```python
from build123d import *

# Parameters (mm, degrees)
SCHIZZO1_W                   = 20
SCHIZZO1_H                   = 20
ESTRUSIONE_ESTRUSIONE1_DEPTH = 58.2
SCHIZZO2_R                   = 2.05
TAGLIO_ESTRUSIONE1_DEPTH     = 60.893572276
FORO_FILETTATO_G1_8_1_D      = 8.8
FORO_FILETTATO_G1_8_1_DEPTH  = 10
FORO_FILETTATO_G1_8_1_TIP    = 2.643786724
M3_TAPPED_HOLE2_D            = 2.5
M3_TAPPED_HOLE2_DEPTH        = 5
M3_TAPPED_HOLE2_TIP          = 0.751075774
M3_TAPPED_HOLE3_REACH        = 60.911
M3_TAPPED_HOLE3_BORE_R       = 1.25
SKETCH1_W                    = 36.2
SKETCH1_H                    = 6
BOSS_EXTRUDE1_DEPTH          = 4.9
CUT_EXTRUDE1_DEPTH           = 65.087830449
M3_TAPPED_HOLE4_D            = 2.5
M3_TAPPED_HOLE4_DEPTH        = 20
M3_TAPPED_HOLE4_TIP          = 0.751075774


with BuildPart() as part:
    # Schizzo1 → Estrusione-Estrusione1 (new body)
    with BuildSketch(Plane.XY):
        Rectangle(SCHIZZO1_W, SCHIZZO1_H)
    extrude(amount=-ESTRUSIONE_ESTRUSIONE1_DEPTH)

    # Schizzo2 → Taglio-Estrusione1 (cut, through all)
    with BuildSketch(Plane(origin=(0, 0, -58.2), x_dir=(-1, 0, 0), z_dir=(0, 0, -1))):
        Circle(SCHIZZO2_R)
    extrude(amount=-TAGLIO_ESTRUSIONE1_DEPTH, mode=Mode.SUBTRACT)

    # Foro filettato G1/8-1
    with Locations(Plane.XY):
        with Locations((0, 0)):
            Hole(FORO_FILETTATO_G1_8_1_D / 2, depth=FORO_FILETTATO_G1_8_1_DEPTH)
            with Locations((0, 0, -(FORO_FILETTATO_G1_8_1_DEPTH + FORO_FILETTATO_G1_8_1_TIP / 2))):  # 118° drill point
                Cone(0, FORO_FILETTATO_G1_8_1_D / 2, FORO_FILETTATO_G1_8_1_TIP, mode=Mode.SUBTRACT)

    # M3 Tapped Hole2
    with Locations(Plane(origin=(0, 10, -29.1), x_dir=(1, 0, 0), z_dir=(0, 1, 0))):
        with Locations((0, 0)):
            Hole(M3_TAPPED_HOLE2_D / 2, depth=M3_TAPPED_HOLE2_DEPTH)
            with Locations((0, 0, -(M3_TAPPED_HOLE2_DEPTH + M3_TAPPED_HOLE2_TIP / 2))):  # 118° drill point
                Cone(0, M3_TAPPED_HOLE2_D / 2, M3_TAPPED_HOLE2_TIP, mode=Mode.SUBTRACT)

    # Schizzo14 → Foro Ø16.0 (16)-1 (revolve, cut)
    with BuildSketch(Plane(origin=(0, 0, -58.2), x_dir=(0, 1, 0), z_dir=(1, 0, 0))):
        Polygon((0, 0), (0, 16.806884952), (8, 12), (8, 0), align=None)
    revolve(axis=Axis((0, 0, -64.55), (0, 0, 1)), mode=Mode.SUBTRACT)

    # M3 Tapped Hole3 bore (on position points) → M3 Tapped Hole3 (cut, up to next)
    with BuildSketch(Plane(origin=(10, 5.5, -53.2), x_dir=(0, 0, 1), z_dir=(1, 0, 0)), mode=Mode.PRIVATE) as m3_tapped_hole3_sk1:
        Circle(M3_TAPPED_HOLE3_BORE_R)
    m3_tapped_hole3_tool1 = extrude(m3_tapped_hole3_sk1.sketch, amount=-M3_TAPPED_HOLE3_REACH, mode=Mode.PRIVATE) & part.part
    # M3 Tapped Hole3 bore (on position points) → M3 Tapped Hole3 (cut, up to next)
    with BuildSketch(Plane(origin=(10, 5.5, -53.2), x_dir=(0, 0, 1), z_dir=(1, 0, 0)), mode=Mode.PRIVATE) as m3_tapped_hole3_sk2:
        with Locations((0, 11)):
            Circle(M3_TAPPED_HOLE3_BORE_R)
    m3_tapped_hole3_tool2 = extrude(m3_tapped_hole3_sk2.sketch, amount=-M3_TAPPED_HOLE3_REACH, mode=Mode.PRIVATE) & part.part
    add(m3_tapped_hole3_tool1.solids().sort_by_distance((10, 5.5, -53.2))[0], mode=Mode.SUBTRACT)
    add(m3_tapped_hole3_tool2.solids().sort_by_distance((10, -5.5, -53.2))[0], mode=Mode.SUBTRACT)

    # Sketch1 → Boss-Extrude1 (add)
    with BuildSketch(Plane.ZY.offset(10)):
        with Locations((-40.1, 0)):
            Rectangle(SKETCH1_W, SKETCH1_H)
    extrude(amount=BOSS_EXTRUDE1_DEPTH)

    # Sketch2 → Cut-Extrude1 (cut, through all)
    with BuildSketch(Plane(origin=(10, 0, 0), x_dir=(0, 0, -1), z_dir=(1, 0, 0))):
        Polygon((50.1, -10), (34.1, -10), (8.1, -10), (8.1, -7), (34.1, -7), (50.1, -7), align=None)
    extrude(amount=-CUT_EXTRUDE1_DEPTH, mode=Mode.SUBTRACT)

    # M3 Tapped Hole4
    with Locations(Plane.XY.offset(-22)):
        with Locations((-13, 0)):
            Hole(M3_TAPPED_HOLE4_D / 2, depth=M3_TAPPED_HOLE4_DEPTH)
            with Locations((0, 0, -(M3_TAPPED_HOLE4_DEPTH + M3_TAPPED_HOLE4_TIP / 2))):  # 118° drill point
                Cone(0, M3_TAPPED_HOLE4_D / 2, M3_TAPPED_HOLE4_TIP, mode=Mode.SUBTRACT)


solid = part.part
```
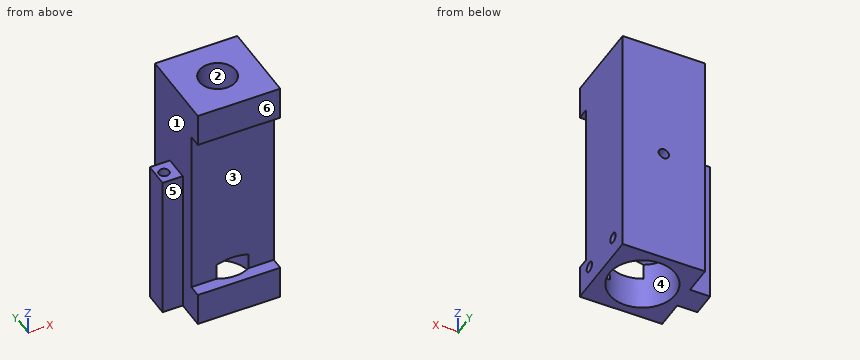
For this review, take the finished solid that the model builds, in its own axes (mm). Face numbers are marked on the shaded views. A direction names the side the tool comes from. Give positions to 0.01 mm unless a question says otherwise; leave off trailing zeros. Write each loop counter-clockwise with the first axis right and the second up, starting at its lowest first coordinate (ties: lowest second). Pieces come first, ordered by that corner, then holes. Notation, with made-up numbers: M -35,54 L -22,54 A23 ccw -22,73 Z; hole C -12.5,43 d9. An arc over 180 degrees is marked long. One line per item, written item: value.
1) For P1, Ø5, axis at x = 5.5, z = -45.5, coming from the -Y side; P2, Ø2, axis at y = -5.5, z = -53.2, coming from the +X side; P3, Ø1.5, axis at x = -11.5, y = -1, coming from the +Z side, all flat-tipped, find the tip position at first contact; note any pin that passes through.
Results are:
P1: stops at y = -7
P2: stops at x = -4.66
P3: stops at z = -22
2) Take a section at B-B, the plane z = -53.2. Write out the cut boundary in (x, y), then the cut area to 3 significant figures.
Results are:
outline: M -14.9,-3 L -10,-3 L -10,-10 L 10,-10 L 10,-6.75 L 4.29,-6.75 A8 cw long 4.29,6.75 L 10,6.75 L 10,10 L -10,10 L -10,3 L -14.9,3 Z; M 6.78,-4.25 L 10,-4.25 L 10,4.25 L 6.78,4.25 A8 cw Z
area: 207 mm²
3) Take a section at A-A, the plane z = -39. Write out the cut boundary in (x, y), then the cut area to 3 significant figures.
Results are:
outline: M -14.9,-3 L -10,-3 L -10,-7 L 10,-7 L 10,10 L -10,10 L -10,3 L -14.9,3 Z; hole C -13,0 d2.5; hole C 0,0 d4.1
area: 351 mm²
4) For the marked faces 4, 5 and 6, list the 3-axis set-ups (+Z, -Z, +X, -X, +Y, -Y) from which the entire face can be reached by the end or side of a thin tool; tool diameter is ignored.
Results are:
face 4: -Z
face 5: +Z, -Z, -X, -Y
face 6: +Z, -Z, +X, -X, -Y
5) For line 1 (X direction, y = 0, z = -33); line 2 (X direction, y = 7.65, z = -29.1); line 3 (Z direction, x = 0.25, y = -9), list the stretches that pass through material, from the lowest coordinate up. Write a range as from..to.
Results are:
line 1: x = -14.9..-14.25, -11.75..-2.05, 2.05..10
line 2: x = -10..-1.25, 1.25..10
line 3: z = -58.2..-50.1, -8.1..0
6) The part is to be moulded in two halves that separate along X. For the marked faces 1, 2 and 3, say which applies: +X half, -X half, draft (parallel to the pull), parting line (faces both ways), or undercut.
Results are:
face 1: -X half
face 2: undercut
face 3: draft
